Input: part model. Units: mm. Frame: model coordinates. A direction names the side the tool comes from. Give positions to 0.01 mm unless a question says otherwise; leave off trailing zeros. Loops run counter-clockwise (first coordinate to the right, second up) from the corner with the lowest first, then second, coordinate; pieces in that order, holes last. Notation, with made-up numbers: M -29,48 L -7,48 A18 ccw -7,61 Z; hole C -13.75,67.5 d8. An arc over 180 degrees is marked long. Use a Markdown table: item, result. Add a question column.
from build123d import *

# Parameters (mm, degrees)
SKETCH1_W           = 35
SKETCH1_H           = 25
BOSS_EXTRUDE1_DEPTH = 24
CUT_EXTRUDE1_DEPTH  = 41.397006939
SKETCH5_R           = 0.95
CUT_EXTRUDE2_DEPTH  = 7


with BuildPart() as part:
    # Sketch1 → Boss-Extrude1 (new body)
    with BuildSketch(Plane(origin=(0, 0, 0), x_dir=(1, 0, 0), z_dir=(0, 1, 0))):
        Rectangle(SKETCH1_W, SKETCH1_H)
    extrude(amount=BOSS_EXTRUDE1_DEPTH)

    # Sketch4 → Cut-Extrude1 (cut, through all)
    with BuildSketch(Plane(origin=(-4.375, -7.577722283, 0), x_dir=(-0.8660254037844417, 0.49999999999999495, 0), z_dir=(-0.49999999999999495, -0.8660254037844417, 0))):
        Polygon((-7.25, 20.405444566), (13.155444566, 0), (-7.25, -20.405444566), (-27.655444566, 0), align=None)
    extrude(amount=-CUT_EXTRUDE1_DEPTH, mode=Mode.SUBTRACT)

    # Sketch5 → Cut-Extrude2 (cut)
    with BuildSketch(Plane.ZY.offset(17.5)):
        with Locations((-10.5, 22)):
            Circle(SKETCH5_R)
        with Locations((10.5, 22)):
            Circle(SKETCH5_R)
        with Locations((10.5, 9.5)):
            Circle(SKETCH5_R)
        with Locations((-10.5, 9.5)):
            Circle(SKETCH5_R)
    extrude(amount=-CUT_EXTRUDE2_DEPTH, mode=Mode.SUBTRACT)


solid = part.part
1) Ray query, line 1 (Y direction, x = -13.25, z = 10.5); line 2 (Z direction, x = -5.5, y = 12.75); line 3 (Z direction, x = -8, y = 3.25). Return the intervals inside material, ascending. Write a range as [from, to].
2) Section query D-D, the plane z = 10.5. Return the cut outline in (x, y).
3) Contact query for flat-ended pins moving along their axis: P1, Ø1.5, axis at y = 22, z = 10.5, coming from the -X side; P2, Ø3, axis at y = 2.5, z = -8, coming from the +X side; P3, Ø1.7, axis at y = 9.5, z = 10.5, coming from the +X side. Output: stop coordinate, or through.
4) Reachability of faces 4 (the flat face through (-13, 0, -3)), 5 (the flat face through (-1.09, 11.74, -6.34)), 6 (the flat face through (-10.5, 22, -11)) from +Z, -Z, +X, -X, +Y, -Y: full face, straight path, thin tool, end or side. Return the list, or none.
5) Section query C-C, the plane x = -9. Return the cut outline in (y, z).
6) Section query A-A, the plane x = 5. Return the cut outline in (y, z), and give its area (3 significant figures).
7) Section query B-B, the plane y = 9.5. Return the cut outline in (x, z).
8) Pull-direction query (Y, two-part tool) for faces 1 (the flat face through (-1.244, 11.832, 6.163)), 2 (the flat face through (-6, 12, 12.5)), 3 (the cylindrical face through (-14.049, 21.073, 10.294)); classes: pulls with the +Y half, pulls with the -Y half, needs draft (parallel to the pull), parting line crosses it, or undercut.
Entries:
| question | item | result |
|---|---|---|
| 1 | line 1 | y = [0, 8.55], [10.45, 21.05], [22.95, 24] |
| 1 | line 2 | z = [-12.5, -2.02], [2.02, 12.5] |
| 1 | line 3 | z = [-12.5, -4.6], [4.6, 12.5] |
| 2 | outline | M -17.5,0 L -3.07,0 L 10.79,24 L -17.5,24 L -17.5,22.95 L -10.5,22.95 L -10.5,21.05 L -17.5,21.05 L -17.5,10.45 L -10.5,10.45 L -10.5,8.55 L -17.5,8.55 Z |
| 3 | P1 | stops at x = -10.5 |
| 3 | P2 | stops at x = -2.57 |
| 3 | P3 | stops at x = 3.52 |
| 4 | face 4 | +Z, -Z, +X, -X, -Y |
| 4 | face 5 | +X, -Y |
| 4 | face 6 | -X |
| 5 | outline | M 0,-12.5 L 24,-12.5 L 24,12.5 L 0,12.5 L 0,5.36 L 10.72,0 L 0,-5.36 Z |
| 6 | outline | M 9.97,-12.5 L 24,-12.5 L 24,-5.49 Z; M 9.97,12.5 L 24,5.49 L 24,12.5 Z |
| 6 | area | 98.4 mm² |
| 7 | outline | M -17.5,-12.5 L 4.73,-12.5 L -9.71,0 L 4.73,12.5 L -17.5,12.5 L -17.5,11.45 L -10.5,11.45 L -10.5,9.55 L -17.5,9.55 L -17.5,-9.55 L -10.5,-9.55 L -10.5,-11.45 L -17.5,-11.45 Z |
| 8 | face 1 | pulls with the -Y half |
| 8 | face 2 | needs draft |
| 8 | face 3 | undercut |
